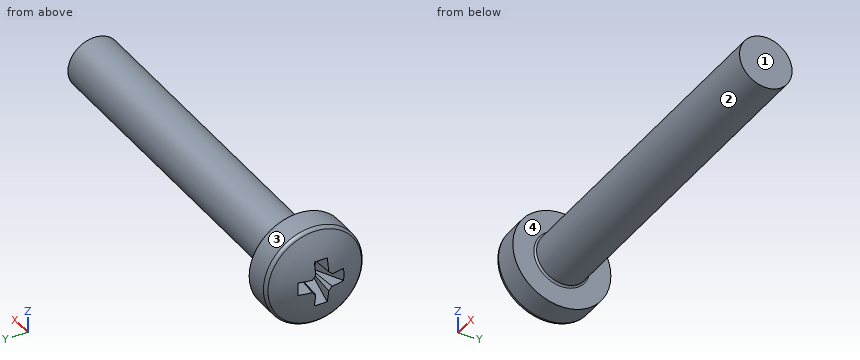
from build123d import *

# Parameters (mm, degrees)
FILLET1_R    = 0.1
SKETCH3_W    = 0.74
SKETCH3_H    = 2.8
SKETCH4_W    = 0.74
SKETCH4_H    = 1.054964432
RECPAT_COUNT = 2
RECPAT_ANGLE = 90


with BuildPart() as part:
    # BodySke → Base-Revolve (revolve)
    with BuildSketch(Plane.XY):
        with BuildLine():
            Line((2.4, 1.5), (2.4, 2.8))
            Line((2.4, 2.8), (1.003501533, 2.8))
            ThreePointArc((1.003501533, 2.8), (0.873295971, 2.76653015), (0.775371599, 2.674418605))
            ThreePointArc((0.775371599, 2.674418605), (0.197753546, 1.392274756), (0, 0))
            Line((0, 0), (22.4, 0))
            Line((22.4, 0), (22.4, 1.5))
            Line((22.4, 1.5), (2.4, 1.5))
        make_face()
    revolve(axis=Axis((-25.4, 0, 0), (1, 0, 0)))

    # Fillet1
    fillet1_edges = [part.edges().sort_by_distance(p)[0] for p in [
        (2.4, -1.5, 0),
    ]]
    fillet(fillet1_edges, radius=FILLET1_R)

    # Sketch3 → Recess section 0
    with BuildSketch(Plane(origin=(0, 0, 0), x_dir=(0, 0, -1), z_dir=(1, 0, 0))):
        Rectangle(SKETCH3_W, SKETCH3_H)
    # Sketch4 → Recess section 1
    with BuildSketch(Plane(origin=(1.75, 0, 0), x_dir=(0, 0, -1), z_dir=(1, 0, 0))):
        Rectangle(SKETCH4_W, SKETCH4_H)
    recess = loft(mode=Mode.SUBTRACT)

    # RecPat: Recess ×2 about axis
    recpat_axis = Axis((0, 0, 0), (1, 0, 0))
    for i in range(1, RECPAT_COUNT):
        add(recess.rotate(recpat_axis, i * RECPAT_ANGLE / (RECPAT_COUNT - 1)), mode=Mode.SUBTRACT)

    # RecCorSke → RecessCore (revolve, cut)
    with BuildSketch(Plane.XY):
        Polygon((0, 0), (0, 0.678371921), (1.75, 0.556), (1.930655351, 0), align=None)
    revolve(axis=Axis((-3.175, 0, 0), (1, 0, 0)), mode=Mode.SUBTRACT)


solid = part.part
Could you check a few things on this model? Use its own coordinates, in mm. Face numbers are marked on the shaded views. A direction names the side the tool comes from. Give positions to 0.01 mm unless a question says otherwise; leave off trailing zeros. Order: outer loops, then holes, each group sorted by start corner. A loop starts at its lowest first (then second) coordinate and runs counter-clockwise, first axis right, second up. Notation, with made-up numbers: (71.25, 17.25) -> (102.25, 17.25) arc R16 cw to (102.25, 30.25) -> close; hole circle Ø9 at (13.5, 60.25). An arc over 180 degrees is marked (long way). Answer in a Markdown table with one row per item. Add a question column.
Item 1: For the marked faces 1 and 2, which set-ups out of +Z, -Z, +X, -X, +Y, -Y let a thin tool reach every point of the face, with its end or its side?
Item 2: Imagine slicing it at A-A (x = 14.25). List the corners of the cut face in (y, z) for me.
Item 3: We'd pull the mould along X, two halves only. Please class the marked faces 3 and 4: pulls with the +X half, pulls with the -X half, needs draft (parallel to the pull), parting line crosses it, or undercut.
Item 4: Please list where these lines run through material, in increasing order: probe 1 along X at (y, z) = (-2.05, 1.05); probe 2 along Z at (x, y) = (21.25, 0.85); probe 3 along Y at (x, z) = (11.5, -1.3).
Item 5: I'm going to push flat-ended pins straight in: P1, Ø1, axis at x = 19.5, y = -1, coming from the +Z side; P2, Ø1.5, axis at x = 12, y = 1.5, coming from the -Z side; P3, Ø2, axis at x = 18.5, z = 2, coming from the +Y side. Where does each tip first touch, or does it pass through?
Result:
| question | item | result |
|---|---|---|
| 1 | face 1 | +Z, -Z, +X, +Y, -Y |
| 1 | face 2 | +X |
| 2 | outline | circle Ø3 at (0, 0) |
| 3 | face 3 | needs draft |
| 3 | face 4 | pulls with the +X half |
| 4 | probe 1 | 0.56 to 2.4 |
| 4 | probe 2 | -1.24 to 1.24 |
| 4 | probe 3 | -0.75 to 0.75 |
| 5 | P1 | z = 1.41 |
| 5 | P2 | z = -1.3 |
| 5 | P3 | y = 1.12 |
